Input: dimensioned drawing with shaded views. Units: mm. Origin: part minimum x, y, z. Give positions to 0.01 mm unless a question says otherwise; leave off trailing zeros. Order: outer loops, then holes, each group sorted by start corner. A loop starts at its lowest first (then second) coordinate and runs counter-clockwise, first axis right, second up. Notation, with made-up numbers: (21.5, 2) - (38.5, 2) arc R22 cw to (38.5, 32) - close; hole circle Ø1 at (73, -36). An arc over 180 degrees is marked (long way). Use a Markdown table: item, result.
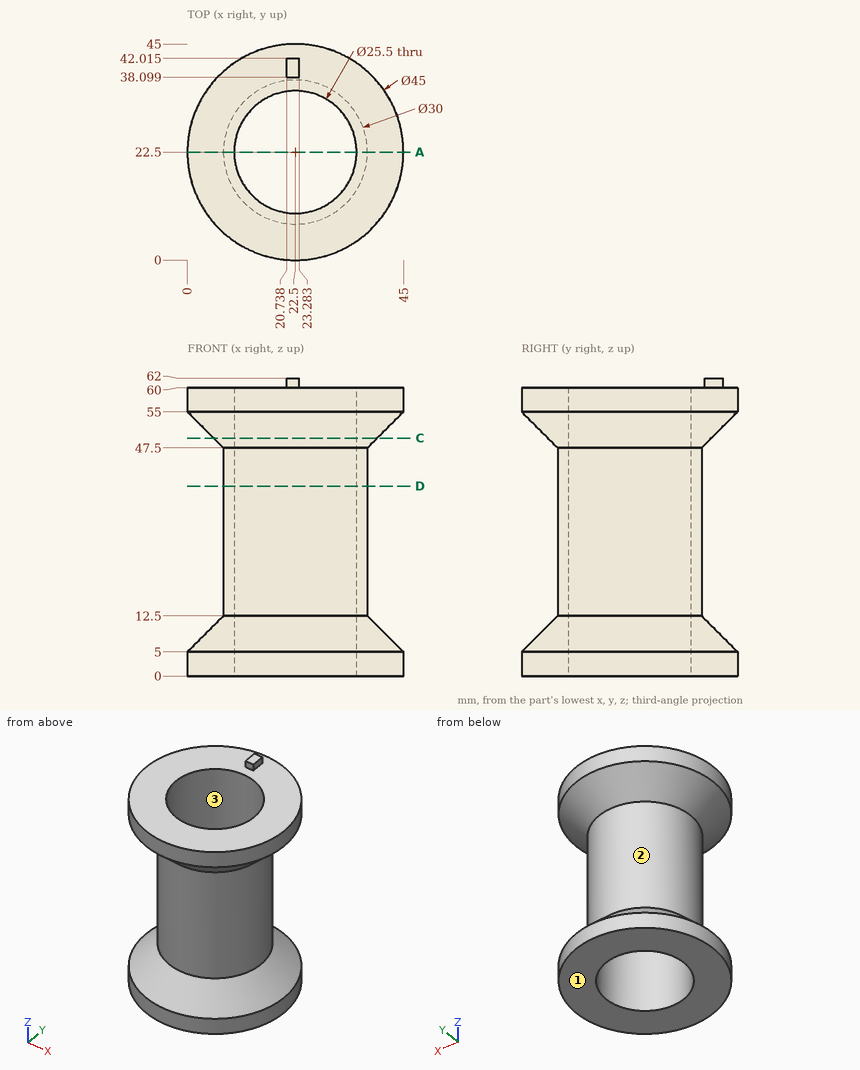
1. Section query A-A (y = 22.5). Return loops of the section in (x, z).
Response:
| item | result |
|---|---|
| outline | (0, 0) - (9.75, 0) - (9.75, 60) - (0, 60) - (0, 55) - (7.5, 47.5) - (7.5, 12.5) - (0, 5) - close; (35.25, 0) - (45, 0) - (45, 5) - (37.5, 12.5) - (37.5, 47.5) - (45, 55) - (45, 60) - (35.25, 60) - close |
2. Section query C-C (z = 49.5). Return loops of the section in (x, y).
Response:
| item | result |
|---|---|
| outline | circle Ø34 at (22.5, 22.5); hole circle Ø25.5 at (22.5, 22.5) |
3. Mould query, pull axis Z, two halves, no side actions, for the marked faces 1, 2 and 3. Classes: pulls with the +Z half, pulls with the -Z half, needs draft (parallel to the pull), parting line crosses it, or undercut.
Response:
| item | result |
|---|---|
| face 1 | pulls with the -Z half |
| face 2 | undercut |
| face 3 | needs draft |
4. Material intervals for line 1 along Y through (x, z) = (22.5, 33); line 2 along X through (y, z) = (24, 20) (1 decimal); line 3 along X through (y, z) = (13.5, 44.5), sorted ascending.
Response:
| item | result |
|---|---|
| line 1 | y = 7.5 to 9.75, 35.25 to 37.5 |
| line 2 | x = 7.6 to 9.8, 35.2 to 37.4 |
| line 3 | x = 10.5 to 13.47, 31.53 to 34.5 |
5. Pin query (flat end, axial travel): pin 1 (5 mm diameter, centred on y = 30.5, z = 33.5, fed in from +X) (1 decimal); pin 2 (2 mm diameter, centred on x = 24, z = 12, fed in from -Y) (1 decimal); pin 3 (1.5 mm diameter, centred on x = 23, z = 44, fed in from -Y). Return the tip coordinate at first contact, or that it passes through.
Response:
| item | result |
|---|---|
| pin 1 | stops at x = 36.5 |
| pin 2 | stops at y = 6.1 |
| pin 3 | stops at y = 7.5 |
6. Section query D-D (z = 39.5). Return loops of the section in (x, y), then the cut area to 3 significant figures.
Response:
| item | result |
|---|---|
| outline | circle Ø30 at (22.5, 22.5); hole circle Ø25.5 at (22.5, 22.5) |
| area | 196 mm^2 |
